The listing builds one solid part. Answer for the finished solid, in the listing's coordinates (mm). Face numbers are marked on the shaded views. A direction names the side the tool comes from. Round coordinates to 2 decimals unless told otherwise and drop trailing zeros. Write each loop counter-clockwise with the first axis right and the second up, starting at its lowest first coordinate (ties: lowest second). Pieces come first, ordered by that corner, then holes. Notation, with made-up numbers: (23.25, 6) - (75.25, 6) arc R23 cw to (75.25, 42) - close; hole circle Ø7 at (76, 53.25). An arc over 180 degrees is marked (long way). Use a Markdown table: item, result. Add a question column.
1) A cutting plane is placed at C-C (z = -3.5). Give the vertices of the cut face in (x, y).
2) Determine the mould class of the marked faces 3, 4 and 5 for opening direction X: +X half, -X half, draft (parallel to the pull), parting line (faces both ways), or undercut.
3) Find the intervals of material crossed by probe 1 along X at (y, z) = (0, -8.5) (3 decimals); probe 2 along X at (y, z) = (0, -6.2); probe 3 along Y at (x, z) = (-3.5, -7), in increasing order. Write a range as from..to.
4) Each of these flat-tipped pins is pushed along its axis until it touches: P1, Ø1.5, axis at y = -3.5, z = -10.5, coming from the +X side; P2, Ø1.5, axis at x = 6.5, z = -6, coming from the +Y side; P3, Ø4, axis at x = -1.5, y = 12, coming from the -Z side (3 decimals). Where does it stop, or does it pass through?
5) A tool of negligible diameter and unlimited length cuts with its end or side. For the marked faces 1 and 2, from which of +Z, -Z, +X, -X, +Y, -Y can it reach the whole face along a straight path? Write none if from no direction.
6) A cutting plane is placed at B-B (z = -5.25). Give the vertices of the cut face in (x, y).
```python
from build123d import *

# Parameters (mm, degrees)
F3_DEPTH  = 9.4615
F6_SIZE   = 1.27
F7_R      = 4.7625
F8_DEPTH  = 5.08
F10_DEPTH = 4.3815


with BuildPart() as f1:
    # F0 (on Right) → F1 (revolve)
    with BuildSketch(Plane.YZ):
        Polygon((0, -14.2875), (0, 0), (-16.51, 0), (-16.51, -9.525), (-12.54125, -9.525), (-12.54125, -6.35), (-9.525, -6.35), (-9.525, -14.2875), align=None)
    revolve(axis=Axis((0, 0, -7.14375), (0, 0, 1)))

    # F2 (on face) → F3 (cut)
    with BuildSketch(Plane(origin=(0, 0, -14.2875), x_dir=(1, 0, 0), z_dir=(0, 0, -1))):
        with BuildLine():
            Line((-1.39492, -1.143), (1.39492, -1.143))
            ThreePointArc((1.39492, -1.143), (0, 1.8034), (-1.39492, -1.143))
        make_face()
    extrude(amount=-F3_DEPTH, mode=Mode.SUBTRACT)

    # F4 (on Right) → F5 (revolve, cut)
    with BuildSketch(Plane.YZ):
        Polygon((-9.525, 0), (-11.90625, 0), (-9.525, -2.38125), align=None)
    revolve(axis=Axis((0, -9.525, -1.190625), (0, 0, -1)), mode=Mode.SUBTRACT)

    # F6
    f6_edges = [f1.edges().sort_by_distance(p)[0] for p in [
        (0, 16.51, 0),
    ]]
    chamfer(f6_edges, length=F6_SIZE)

    # F7 (on face) → F8 (cut)
    with BuildSketch(Plane(origin=(0, 0, -14.2875), x_dir=(1, 0, 0), z_dir=(0, 0, -1))):
        Circle(F7_R)
    extrude(amount=-F8_DEPTH, mode=Mode.SUBTRACT)

    # F9 (on face) → F10 (cut, through all)
    with BuildSketch(Plane(origin=(0, 0, -9.2075), x_dir=(1, 0, 0), z_dir=(0, 0, -1))):
        with BuildLine():
            Line((-1.430541, -1.2192), (1.430541, -1.2192))
            ThreePointArc((1.430541, -1.2192), (0, 1.8796), (-1.430541, -1.2192))
        make_face()
    extrude(amount=-F10_DEPTH, mode=Mode.SUBTRACT)


solid = f1.part
```
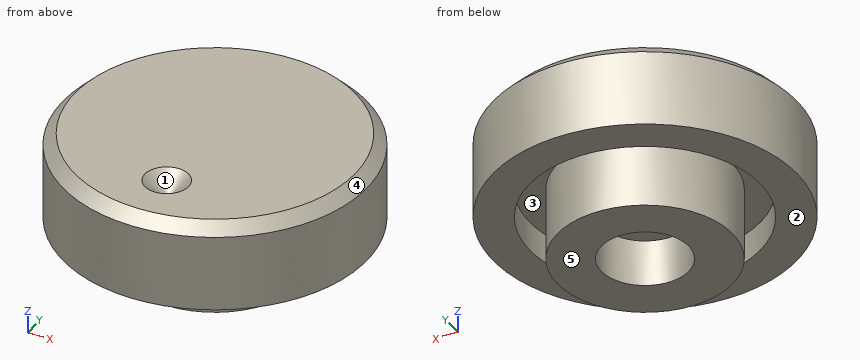
Entries:
| question | item | result |
|---|---|---|
| 1 | outline | circle Ø33.02 at (0, 0) |
| 2 | face 3 | undercut |
| 2 | face 4 | parting line |
| 2 | face 5 | draft |
| 3 | probe 1 | x = -16.51..-12.541, -9.525..-1.88, 1.88..9.525, 12.541..16.51 |
| 3 | probe 2 | x = -16.51..-1.88, 1.88..16.51 |
| 3 | probe 3 | y = -16.13..-12.04, -8.86..8.86, 12.04..16.13 |
| 4 | P1 | stops at x = 9.12 |
| 4 | P2 | stops at y = 15.48 |
| 4 | P3 | stops at z = -9.525 |
| 5 | face 1 | +Z |
| 5 | face 2 | -Z |
| 6 | outline | circle Ø33.02 at (0, 0); hole (-1.43, 1.22) arc R1.88 ccw (long way) to (1.43, 1.22) - close |
